Model file for the job. Use its own axes, mm. Give positions to 0.01 mm unless a question says otherwise; leave off trailing zeros. Order: outer loops, then holes, each group sorted by start corner. A loop starts at its lowest first (then second) coordinate and runs counter-clockwise, first axis right, second up. Notation, with made-up numbers: M -34.75,2.25 L 16.25,2.25 A20 cw 16.25,17.25 Z; hole C -2,55.5 d10. An arc over 180 degrees is marked long. Return JSON: item names as keys, results as strings. Group by question number.
1. Slice it at B-B on y = 19.5. List the corners of the cut face in (x, z), then the cut area to 3 significant figures.
2. Wall check: probe 1 along Z at (x, y) = (-8, 10.75); probe 2 along Z at (x, y) = (-2.5, 15); probe 3 along Y at (x, z) = (-20.5, 26). Give the ranges that are in metal, low to high. Write a range as [from, to].
3. Slice it at C-C on z = -24.5. List the corners of the cut face in (x, y), then the cut area to 3 significant figures.
4. Pin check, flat tips, straight feed: pin 1 (8 mm diameter, centred on x = 21, y = 13.5, fed in from +Z); pin 2 (6 mm diameter, centred on x = 23.5, y = 18, fed in from +Z). Stop position of each tip, or through.
from build123d import *

# Parameters (mm, degrees)
SKETCH_1_W      = 70
SKETCH_1_H      = 60
EXTRUDE_1_DEPTH = 22
FILLET_1_R      = 11


with BuildPart() as part:
    # 草图1 → 凸台-拉伸1 (new body)
    with BuildSketch(Plane(origin=(0, 0, 0), x_dir=(1, 0, 0), z_dir=(0, 1, 0))):
        Rectangle(SKETCH_1_W, SKETCH_1_H)
    extrude(amount=EXTRUDE_1_DEPTH)

    # 圆角1
    fillet_1_edges = [part.edges().sort_by_distance(p)[0] for p in [
        (0, 0, -30),
        (0, 22, -30),
        (0, 0, 30),
        (0, 22, 30),
    ]]
    fillet(fillet_1_edges, radius=FILLET_1_R - 0.0001)  # a hair under: the kernel refuses the full size


solid = part.part
Result:
{
 "1": {"outline": "M -35,-25.98 L 35,-25.98 L 35,25.98 L -35,25.98 Z", "area": "3,640 mm2"},
 "2": {"probe 1": "z = [-30, 30]", "probe 2": "z = [-29.25, 29.25]", "probe 3": "y = [2.51, 19.49]"},
 "3": {"outline": "M -35,1.47 L 35,1.47 L 35,20.53 L -35,20.53 Z", "area": "1,330 mm2"},
 "4": {"pin 1": "stops at z = 30", "pin 2": "stops at z = 29.25"}
}
